Build history of the part. All positions in model axes, mm. Coordinates: 2 decimals unless noted, no trailing zeros. Loops run counter-clockwise (first coordinate to the right, second up) from the corner with the lowest first, then second, coordinate; pieces in that order, holes last.
Item 1: Cut at C-C (x = 57). List the corners of the cut face in (y, z), and give its area (3 significant figures).
Item 2: Cut at B-B (z = 0). List the corners of the cut face in (x, y).
Item 3: Flat gauge pin, fed straight in: pin 1 (3 mm diameter, centred on x = 9.5, y = 37.5, fed in from -Z). Where does the tip first touch, or does it go through?
Item 4: Cut at A-A (y = 17.5). List the corners of the cut face in (x, z), and give its area (3 significant figures).
Item 5: Drill centre lines: line 1 along X through (y, z) = (11, -0.1); line 2 along X through (y, z) = (27, -0.45); line 3 along Y through (x, z) = (25, -0.35). Where is each one in solid material? Low to high.
from build123d import *

# Parameters (mm, degrees)
F1_R = 0.6515882549


with BuildPart() as f2:
    # F2: sweep along a path in F0
    with BuildLine(Plane.XY) as f2_path:
        Line((0, 0), (0, 28.2141789794))
        Line((0, 28.2141789794), (26.0536126347, 43.2562392474))
        Line((26.0536126347, 43.2562392474), (62.7735159846, 43.2562392474))
        Line((62.7735159846, 43.2562392474), (87.544889414, 28.9544801298))
        Line((87.544889414, 28.9544801298), (87.544889414, 0))
    # F1 (on Front) → F2 (sweep)
    with BuildSketch(Plane.XZ):
        Circle(F1_R)
    sweep(path=f2_path.line, transition=Transition.RIGHT)


solid = f2.part
Filled sheet:
1. outline: circle Ø1.3 at (43.26, 0)
1. area: 1.33 mm2
2. outline: (-0.65, 0) - (0.65, 0) - (0.65, 27.84) - (26.23, 42.6) - (62.6, 42.6) - (86.89, 28.58) - (86.89, 0) - (88.2, 0) - (88.2, 29.33) - (62.95, 43.91) - (25.88, 43.91) - (-0.65, 28.59) - close
3. pin 1: passes through
4. outline: circle Ø1.3 at (0, 0); circle Ø1.3 at (87.54, 0)
4. area: 2.67 mm2
5. line 1: x = -0.64 to 0.64, 86.9 to 88.19
5. line 2: x = -0.47 to 0.47, 87.07 to 88.02
5. line 3: y = 42.01 to 43.28
